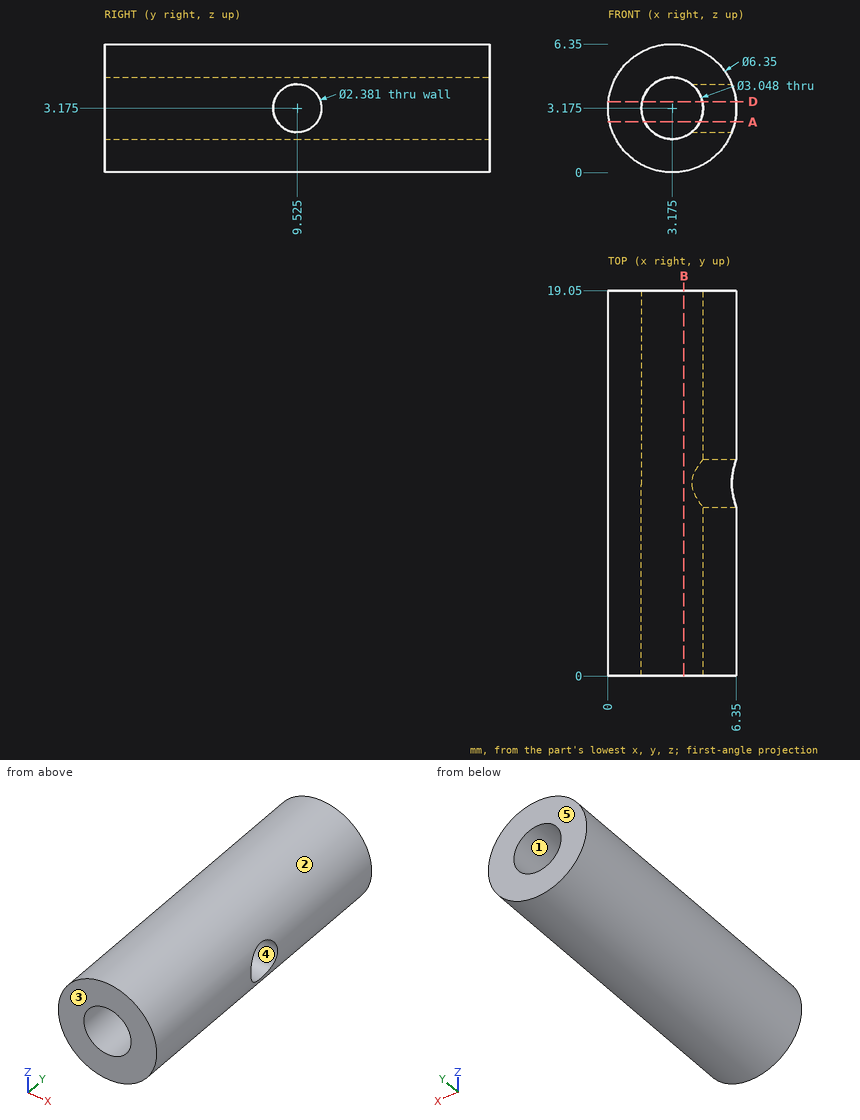
Geometry: see drawing. Coordinates: mm, zero at the bounding-box minimum. A direction names the side the tool comes from. Round coordinates to 2 decimals unless told otherwise and drop trailing zeros. Write each loop counter-clockwise with the first axis right and the second up, starting at its lowest first coordinate (ties: lowest second). Pieces come first, ordered by that corner, then holes.
1) Contact query for flat-ended pins moving along their axis: P1, Ø2, axis at y = 16, z = 1.5, coming from the +X side; P2, Ø1.5, axis at x = 4, y = 5.5, coming from the +Z side. Output: stop coordinate, or through.
2) Cut plane D-D (z = 3.5). Return the cut outline in (x, y).
3) Ray query, L1, parallel to Y at x = 4.75, z = 3.25; L2, parallel to X at y = 17.5, z = 2.25 (1 decimal); L3, parallel to Z at x = 4, y = 13.75. Return the intervals inside material, ascending.
4) Draft query along X for the marked faces 1, 2 and 3. Return one class per face: pulls with the +X half, pulls with the -X half, needs draft (parallel to the pull), parting line crosses it, or undercut.
5) Cut plane A-A (z = 2.5). Return the cut outline in (x, y).
6) Reachability of the marked faces 4 and 5 from +Z, -Z, +X, -X, +Y, -Y: full face, straight path, thin tool, end or side. Return the list, or none.
7) Cut plane B-B (x = 3.75). Return the cut outline in (y, z), then the cut area to 3 significant figures.
Geometry says:
1. P1: stops at x = 6.28
1. P2: stops at z = 6.35
2. outline: (0.02, 0) - (1.69, 0) - (1.69, 19.05) - (0.02, 19.05) - close; (4.66, 0) - (6.33, 0) - (6.33, 8.38) - (4.66, 8.38) - close; (4.66, 10.67) - (6.33, 10.67) - (6.33, 19.05) - (4.66, 19.05) - close
3. L1: y = 0 to 8.34, 10.71 to 19.05
3. L2: x = 0.1 to 2, 4.4 to 6.2
3. L3: z = 0.11 to 1.89, 4.46 to 6.24
4. face 1: undercut
4. face 2: parting line crosses it
4. face 3: needs draft
5. outline: (0.07, 0) - (1.81, 0) - (1.81, 19.05) - (0.07, 19.05) - close; (4.54, 0) - (6.28, 0) - (6.28, 8.54) - (4.54, 8.54) - close; (4.54, 10.51) - (6.28, 10.51) - (6.28, 19.05) - (4.54, 19.05) - close
6. face 4: +X
6. face 5: +Z, -Z, +X, -X, +Y
7. outline: (0, 0.05) - (19.05, 0.05) - (19.05, 1.76) - (0, 1.76) - close; (0, 4.59) - (19.05, 4.59) - (19.05, 6.3) - (0, 6.3) - close
7. area: 65.2 mm2
